from build123d import *

# Parameters (mm, degrees)
SKETCH1_W               = 23.5
SKETCH1_H               = 11
BOSS_EXTRUDE1_DEPTH     = 2.5
BOSS_EXTRUDE2_DEPTH     = 2.5
BOSS_EXTRUDE3_DEPTH     = 13.5
BOSS_EXTRUDE4_DEPTH     = 1
CUT_EXTRUDE1_DEPTH      = 12
SKETCH7_W               = 16
SKETCH7_H               = 2
CUT_EXTRUDE2_DEPTH      = 32.198958316
SKETCH8_R               = 1.375
CUT_EXTRUDE3_DEPTH      = 12
CUT_EXTRUDE5_DEPTH      = 1.5
SKETCH10_R              = 3.5
BOSS_EXTRUDE5_DEPTH     = 2.5
CUT_EXTRUDE6_DEPTH      = 29.34387059
CUT_EXTRUDE6_DEPTH_BACK = 29.34387059
SKETCH11_R              = 1.25


with BuildPart() as part:
    # Sketch1 → Boss-Extrude1 (new body)
    with BuildSketch(Plane(origin=(0, 0, 0), x_dir=(1, 0, 0), z_dir=(0, 1, 0))):
        Rectangle(SKETCH1_W, SKETCH1_H)
    extrude(amount=BOSS_EXTRUDE1_DEPTH)

    # Sketch2 → Boss-Extrude2 (add)
    with BuildSketch(Plane(origin=(0, 2.5, 0), x_dir=(1, 0, 0), z_dir=(0, 1, 0))):
        with BuildLine():
            Line((21.231385291, -3.171040463), (14.511908348, -6.310115609))
            ThreePointArc((14.511908348, -6.310115609), (12.447193964, -7.012201496), (10.279378945, -7.25))
            Line((10.279378945, -7.25), (-10.279378945, -7.25))
            ThreePointArc((-10.279378945, -7.25), (-12.447193964, -7.012201496), (-14.511908348, -6.310115609))
            Line((-14.511908348, -6.310115609), (-21.231385291, -3.171040463))
            ThreePointArc((-21.231385291, -3.171040463), (-23.25, 0), (-21.231385291, 3.171040463))
            Line((-21.231385291, 3.171040463), (-14.511908348, 6.310115609))
            ThreePointArc((-14.511908348, 6.310115609), (-12.447193964, 7.012201496), (-10.279378945, 7.25))
            Line((-10.279378945, 7.25), (10.279378945, 7.25))
            ThreePointArc((10.279378945, 7.25), (12.447193964, 7.012201496), (14.511908348, 6.310115609))
            Line((14.511908348, 6.310115609), (21.231385291, 3.171040463))
            ThreePointArc((21.231385291, 3.171040463), (23.25, 0), (21.231385291, -3.171040463))
        make_face()
    extrude(amount=BOSS_EXTRUDE2_DEPTH)

    # Sketch3 → Boss-Extrude3 (add)
    with BuildSketch(Plane(origin=(0, 5, 0), x_dir=(1, 0, 0), z_dir=(0, 1, 0))):
        Polygon((8.75, -4.75), (3.5, -4.75), (3.5, -6.25), (-3.5, -6.25), (-3.5, -4.75), (-8.75, -4.75), (-11.75, -1.75), (-11.75, 1.75), (-8.75, 4.75), (8.75, 4.75), (11.75, 1.75), (11.75, -1.75), align=None)
    extrude(amount=BOSS_EXTRUDE3_DEPTH)

    # Sketch5 → Boss-Extrude4 (add)
    with BuildSketch(Plane(origin=(0, 18.5, 0), x_dir=(1, 0, 0), z_dir=(0, 1, 0))):
        Polygon((8.75, 4.75), (8.05, 4.75), (8.05, -4.75), (8.75, -4.75), (9.55, -3.95), (9.55, 3.95), align=None)
        Polygon((-8.05, 4.75), (-8.75, 4.75), (-9.55, 3.95), (-9.55, -3.95), (-8.75, -4.75), (-8.05, -4.75), align=None)
    extrude(amount=BOSS_EXTRUDE4_DEPTH)

    # Sketch6 → Cut-Extrude1 (cut)
    with BuildSketch(Plane(origin=(0, 0, 0), x_dir=(1, 0, 0), z_dir=(0, 1, 0))):
        Polygon((8.4, 3.45), (5.1, 3.45), (4.6, 2.95), (4.1, 2.95), (3.6, 3.45), (-3.6, 3.45), (-4.1, 2.95), (-4.6, 2.95), (-5.1, 3.45), (-8.4, 3.45), (-10.35, 1.5), (-10.35, -1.5), (-8.4, -3.45), (-2.05, -3.45), (-2.05, -4.55), (2.05, -4.55), (2.05, -3.45), (8.4, -3.45), (10.35, -1.5), (10.35, 1.5), align=None)
    extrude(amount=CUT_EXTRUDE1_DEPTH, mode=Mode.SUBTRACT)

    # Sketch7 → Cut-Extrude2 (cut, through all)
    with BuildSketch(Plane(origin=(0, 0, 0), x_dir=(1, 0, 0), z_dir=(0, 1, 0))):
        Rectangle(SKETCH7_W, SKETCH7_H)
    extrude(amount=CUT_EXTRUDE2_DEPTH, mode=Mode.SUBTRACT)

    # Sketch8 → Cut-Extrude3 (cut)
    with BuildSketch(Plane.XY.offset(6.25)):
        with Locations((0.625, 15)):
            Circle(SKETCH8_R)
    extrude(amount=-CUT_EXTRUDE3_DEPTH, mode=Mode.SUBTRACT)

    # Sketch9 → Cut-Extrude5 (cut)
    with BuildSketch(Plane.XY.offset(6.25)):
        with BuildLine():
            Line((0.625, 12), (3.5, 12))
            Line((3.5, 12), (3.5, 18.5))
            Line((3.5, 18.5), (-3.5, 18.5))
            Line((-3.5, 18.5), (-3.5, 15))
            Line((-3.5, 15), (-2.375, 15))
            ThreePointArc((-2.375, 15), (-1.496320344, 12.878679656), (0.625, 12))
        make_face()
    extrude(amount=-CUT_EXTRUDE5_DEPTH, mode=Mode.SUBTRACT)

    # Sketch10 → Boss-Extrude5 (add)
    with BuildSketch(Plane(origin=(0, 5, 0), x_dir=(1, 0, 0), z_dir=(0, 1, 0))):
        with Locations(Location((-19.75, 0, 0), (0, 0, 115.040130233))):
            Circle(SKETCH10_R)
        with Locations(Location((19.75, 0, 0), (0, 0, 64.959869767))):
            Circle(SKETCH10_R)
    extrude(amount=BOSS_EXTRUDE5_DEPTH)

    # Sketch11 → Cut-Extrude6 (cut, two sides: drawn at the far end of the back side and taken through both)
    with BuildSketch(Plane(origin=(0, 5, 0), x_dir=(1, 0, 0), z_dir=(0, 1, 0)).offset(-CUT_EXTRUDE6_DEPTH_BACK)):
        with Locations(Location((19.75, 0, 0), (0, 0, 270))):
            Circle(SKETCH11_R)
        with Locations(Location((-19.75, 0, 0), (0, 0, 270))):
            Circle(SKETCH11_R)
    extrude(amount=CUT_EXTRUDE6_DEPTH + CUT_EXTRUDE6_DEPTH_BACK, mode=Mode.SUBTRACT)


solid = part.part
Source: CAD feature listing. Evaluate the final solid. Frame: model axes, mm. A direction names the side the tool comes from. Round coordinates to 2 decimals unless told otherwise and drop trailing zeros. Loops run counter-clockwise (first coordinate to the right, second up) from the corner with the lowest first, then second, coordinate; pieces in that order, holes last. Notation, with made-up numbers: M 76,14.5 L 94,14.5 A26 ccw 94,48.5 Z; hole C 48,-25.5 d2. An arc over 180 degrees is marked long. Return JSON: item names as keys, results as strings. Group by question number.
1. Pin query (flat end, axial travel): pin 1 (1 mm diameter, centred on y = 9, z = 1, fed in from +X); pin 2 (1.2 mm diameter, centred on x = -3, z = 5.5, fed in from +Y); pin 3 (0.8 mm diameter, centred on x = 1.5, z = 5.5, fed in from +Y). Return the tip coordinate at first contact, or that it passes through.
2. Mould query, pull axis Z, two halves, no side actions, for faces 5 (the face through (0, 1, 5.5)), 6 (the face through (0, 17, -1)), 7 (the face through (-9, 19.5, 0)), 8 (the face through (-12.5, 3.7, -7)). Classes: released by +Z, released by -Z, zero draft, split by the parting line, or undercut.
3. Reachability of faces 1 (the face through (8, 15, 0)), 2 (the face through (9.55, 19, 0)), 3 (the face through (-9.36, 5.92, -2.49)), 4 (the face through (-3, 15, 6)) from +Z, -Z, +X, -X, +Y, -Y: full face, straight path, thin tool, end or side. Return the list, or none.
4. Section query C-C on y = 3.5. State how many separate pieces and enclosed holes the cut face has, and give its area (3 significant figures).
5. Section query B-B on x = 19.75. Output: boundary loops of the cut face in (y, z), and give its area (3 significant figures).
6. Material intervals for line 1 along X through (y, z) = (5.05, 0); line 2 along Z through (x, y) = (-6, 2.75); line 3 along Z through (x, y) = (3.5, 16.75), sorted ascending. Write a range as from..to.
Checks:
{
 "1": {"pin 1": "stops at x = 11.75", "pin 2": "stops at y = 15", "pin 3": "stops at y = 12"},
 "2": {"face 5": "released by +Z", "face 6": "undercut", "face 7": "zero draft", "face 8": "released by -Z"},
 "3": {"face 1": "+Y, -Y", "face 2": "+Z, -Z, +X, +Y", "face 3": "-Y", "face 4": "+Z, +X, -X, +Y"},
 "4": {"separate pieces": "1", "enclosed holes": "3", "area": "413 mm²"},
 "5": {"outline": "M 2.5,-3.86 L 5,-3.86 L 5,-3.5 L 7.5,-3.5 L 7.5,-1.25 L 2.5,-1.25 Z; M 2.5,1.25 L 7.5,1.25 L 7.5,3.5 L 5,3.5 L 5,3.86 L 2.5,3.86 Z", "area": "24.3 mm²"},
 "6": {"line 1": "x = -23.25..-21, -18.5..-16.25, -11.75..-10.35, 10.35..11.75, 16.25..18.5, 21..23.25", "line 2": "z = -7.25..-3.45, 3.45..7.25", "line 3": "z = -4.75..-1, 1..4.75"}
}
